For this review, take the finished solid that the model builds, in its own axes (mm). A direction names the side the tool comes from. Coordinates: 2 decimals unless noted, no trailing zeros. Write each loop counter-clockwise with the first axis right and the second up, starting at its lowest first coordinate (ties: lowest second). Pieces come first, ordered by that corner, then holes.
1) To check wall thickness, follow line 1 along Z through (x, y) = (-7.25, 0.5); line 2 along Z through (x, y) = (5.5, 7); line 3 along Y through (x, z) = (-3.5, 2.5). State the ranges of each line that lie inside material, in increasing order.
2) We need section A-A on y = 4. Write out the cut boundary in (x, z).
3) We need section D-D on y = -4.5. Write out the cut boundary in (x, z).
4) Insertion check: P1, Ø8, axis at x = -5, z = -4, coming from the +Y side; P2, Ø1.9, axis at x = -7.34, z = 1.53, coming from the -Y side; P3, Ø7.5, axis at x = 4.5, z = 0, coming from the +Y side. Each pin has a flat end and moves straight along its axis. Give the tip position at first contact, or say it passes through.
5) For faces 1 (the face through (6, 2, 1)), 2 (the face through (-3.018, 5.465, 10.977)), 3 (the face through (3, 8, -7)), list the 3-axis set-ups (+Z, -Z, +X, -X, +Y, -Y) from which the entire face can be reached by the end or side of a thin tool; tool diameter is ignored.
6) Mouldability with a two-part tool opening along Z and no side actions: class faces 4 (the face through (-1, -14, 2)), 5 (the face through (-1, -3, 11.526)), 6 (the face through (6, 5, 8.026)) as pulls with the +Z half, pulls with the -Z half, needs draft (parallel to the pull), parting line crosses it, or undercut.
7) We need section C-C on x = 3.25. Write out the cut boundary in (y, z), then the cut area to 3 significant figures.
8) We need section B-B on z = 0.5. Write out the cut boundary in (x, y), then the cut area to 3 significant figures.
from build123d import *

# Parameters (mm, degrees)
CROQUIS2_W              = 20
CROQUIS2_H              = 20
SALIENTE_EXTRUIR1_DEPTH = 8
CROQUIS3_W              = 6.705751287
CROQUIS3_H              = 13
CORTAR_EXTRUIR1_DEPTH   = 6
CORTAR_EXTRUIR2_DEPTH   = 5
CROQUIS6_R              = 1.6
CORTAR_EXTRUIR3_DEPTH   = 3
REDONDEO1_R             = 1
CROQUIS7_R              = 1.6
SALIENTE_EXTRUIR2_DEPTH = 14


with BuildPart() as part:
    # Croquis2 → Saliente-Extruir1 (new body)
    with BuildSketch(Plane(origin=(0, 0, 0), x_dir=(1, 0, 0), z_dir=(0, 1, 0))):
        with Locations((-0.843373494, -1.526104418)):
            Rectangle(CROQUIS2_W, CROQUIS2_H)
    extrude(amount=SALIENTE_EXTRUIR1_DEPTH)

    # Croquis3 → Cortar-Extruir1 (cut)
    with BuildSketch(Plane(origin=(0, 8, 0), x_dir=(1, 0, 0), z_dir=(0, 1, 0))):
        with Locations((5.803750863, -1.526104418)):
            Rectangle(CROQUIS3_W, CROQUIS3_H)
    extrude(amount=-CORTAR_EXTRUIR1_DEPTH, mode=Mode.SUBTRACT)

    # Croquis5 → Cortar-Extruir2 (cut)
    with BuildSketch(Plane(origin=(0, 8, 0), x_dir=(1, 0, 0), z_dir=(0, 1, 0))):
        with BuildLine():
            Line((2.450875219, -7.526104418), (2.450875219, 4.473895582))
            ThreePointArc((2.450875219, 4.473895582), (2.020425803, 4.459111389), (1.589976387, 4.473895582))
            ThreePointArc((1.589976387, 4.473895582), (-1.703861847, 5.684131739), (-3.832537389, 8.473895582))
            Line((-3.832537389, 8.473895582), (-10.843373494, 8.473895582))
            Line((-10.843373494, 8.473895582), (-10.843373494, -11.526104418))
            Line((-10.843373494, -11.526104418), (-3.832537389, -11.526104418))
            ThreePointArc((-3.832537389, -11.526104418), (-1.703861847, -8.736340574), (1.589976387, -7.526104418))
            ThreePointArc((1.589976387, -7.526104418), (2.020425803, -7.511320225), (2.450875219, -7.526104418))
        make_face()
    extrude(amount=-CORTAR_EXTRUIR2_DEPTH, mode=Mode.SUBTRACT)

    # Croquis6 → Cortar-Extruir3 (cut)
    with BuildSketch(Plane(origin=(0, 3, 0), x_dir=(1, 0, 0), z_dir=(0, 1, 0))):
        with Locations(Location((-7.343373494, -1.526104418, 0), (0, 0, 270))):
            Circle(CROQUIS6_R)
    extrude(amount=-CORTAR_EXTRUIR3_DEPTH, mode=Mode.SUBTRACT)

    # Redondeo1
    redondeo1_edges = [part.edges().sort_by_distance(p)[0] for p in [
        (-10.843373494, 1.5, -8.473895582),
        (-10.843373494, 1.5, 11.526104418),
        (-3.832537389, 5.5, 11.526104418),
        (-3.832537389, 5.5, -8.473895582),
        (9.156626506, 4, -8.473895582),
        (9.156626506, 4, 11.526104418),
    ]]
    fillet(redondeo1_edges, radius=REDONDEO1_R)

    # Croquis7 → Saliente-Extruir2 (add)
    with BuildSketch(Plane.XZ):
        with BuildLine():
            Line((-9.843373494, -8.473895582), (8.156626506, -8.473895582))
            ThreePointArc((8.156626506, -8.473895582), (8.863733287, -8.181002364), (9.156626506, -7.473895582))
            Line((9.156626506, -7.473895582), (9.156626506, 10.526104418))
            ThreePointArc((9.156626506, 10.526104418), (8.863733287, 11.233211199), (8.156626506, 11.526104418))
            Line((8.156626506, 11.526104418), (-9.843373494, 11.526104418))
            ThreePointArc((-9.843373494, 11.526104418), (-10.550480275, 11.233211199), (-10.843373494, 10.526104418))
            Line((-10.843373494, 10.526104418), (-10.843373494, -7.473895582))
            ThreePointArc((-10.843373494, -7.473895582), (-10.550480275, -8.181002364), (-9.843373494, -8.473895582))
        make_face()
        with Locations(Location((-7.343373494, 1.526104418, 0), (0, 0, 90))):
            Circle(CROQUIS7_R, mode=Mode.SUBTRACT)
    extrude(amount=SALIENTE_EXTRUIR2_DEPTH)


solid = part.part
Result:
1. line 1: z = -8.47 to -0.07, 3.12 to 11.53
1. line 2: z = -8.47 to -4.97, 8.03 to 11.53
1. line 3: y = -14 to 3
2. outline: (-2.91, -6.86) arc R1 ccw to (-2.13, -8.47) - (8.16, -8.47) arc R1 ccw to (9.16, -7.47) - (9.16, -4.97) - (2.45, -4.97) - (2.45, -4.47) arc R6.27 ccw to start; (-2.91, 9.91) arc R6.27 ccw to (2.45, 7.53) - (2.45, 8.03) - (9.16, 8.03) - (9.16, 10.53) arc R1 ccw to (8.16, 11.53) - (-2.13, 11.53) arc R1 ccw to start
3. outline: (-10.84, -7.47) arc R1 ccw to (-9.84, -8.47) - (8.16, -8.47) arc R1 ccw to (9.16, -7.47) - (9.16, 10.53) arc R1 ccw to (8.16, 11.53) - (-9.84, 11.53) arc R1 ccw to (-10.84, 10.53) - close; hole circle Ø3.2 at (-7.34, 1.53)
4. P1: stops at y = 8
4. P2: passes through
4. P3: stops at y = 3
5. face 1: +X, +Y
5. face 2: -X, +Y
5. face 3: +Z, -Z, +X, -X, +Y
6. face 4: needs draft
6. face 5: pulls with the +Z half
6. face 6: undercut
7. outline: (-14, -8.47) - (8, -8.47) - (8, -4.97) - (2, -4.97) - (2, 8.03) - (8, 8.03) - (8, 11.53) - (-14, 11.53) - close
7. area: 362 mm2
8. outline: (-10.84, -14) - (-8.57, -14) - (-8.57, 3) - (-10.84, 3) - close; (-6.12, -14) - (9.16, -14) - (9.16, 2) - (2.45, 2) - (2.45, 3) - (-6.12, 3) - close
8. area: 292 mm2
